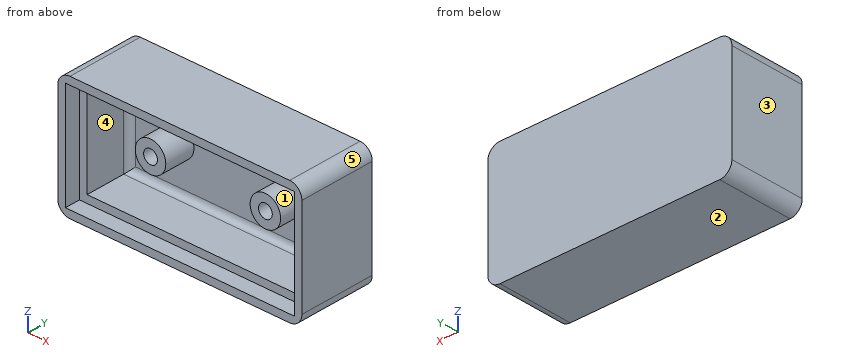
```python
from build123d import *

# Parameters (mm, degrees)
F0_W     = 50.8
F0_H     = 25.4
F0_W_2   = 44.45
F0_H_2   = 19.05
F1_DEPTH = 12.7
F2_W     = 44.45
F2_H     = 19.05
F3_DEPTH = 9.525
F4_R     = 1.27
F5_W     = 50.8
F5_H     = 25.4
F5_W_2   = 47.625
F5_H_2   = 22.225
F6_DEPTH = 3.175
F7_R     = 2.54
F8_R     = 3.175
F8_R_2   = 1.43697608
F9_DEPTH = 6.35


with BuildPart() as f1:
    # F0 (on Front) → F1 (new body)
    with BuildSketch(Plane.XZ):
        Rectangle(F0_W, F0_H)
        Rectangle(F0_W_2, F0_H_2, mode=Mode.SUBTRACT)
        Rectangle(F0_W_2, F0_H_2)
    extrude(amount=F1_DEPTH)

    # F2 (on face) → F3 (cut)
    with BuildSketch(Plane.XZ.offset(12.7)):
        Rectangle(F2_W, F2_H)
    extrude(amount=-F3_DEPTH, mode=Mode.SUBTRACT)

    # F4
    f4_edges = [f1.edges().sort_by_distance(p)[0] for p in [
        (22.225, -3.175, 0),
        (0, -3.175, 9.525),
        (-22.225, -3.175, 0),
        (0, -3.175, -9.525),
    ]]
    fillet(f4_edges, radius=F4_R)

    # F5 (on face) → F6 (join)
    with BuildSketch(Plane.XZ.offset(12.7)):
        Rectangle(F5_W, F5_H)
        Rectangle(F5_W_2, F5_H_2, mode=Mode.SUBTRACT)
    extrude(amount=F6_DEPTH)

    # F7
    f7_edges = [f1.edges().sort_by_distance(p)[0] for p in [
        (25.4, -7.9375, 12.7),
        (25.4, -7.9375, -12.7),
        (-25.4, -7.9375, -12.7),
        (-25.4, -7.9375, 12.7),
    ]]
    fillet(f7_edges, radius=F7_R)

    # F8 (on face) → F9 (join)
    with BuildSketch(Plane.XZ.offset(3.175)):
        with Locations((11.9508895849, 0)):
            Circle(F8_R)
        with Locations((11.9508895849, 0)):
            Circle(F8_R_2, mode=Mode.SUBTRACT)
        with Locations((-11.9508895849, 0)):
            Circle(F8_R)
        with Locations((-11.9508895849, 0)):
            Circle(F8_R_2, mode=Mode.SUBTRACT)
    extrude(amount=F9_DEPTH)


solid = f1.part
```
Work out the finished part from the listing and answer in its coordinate system (mm). Face numbers are marked on the shaded views. A direction names the side the tool comes from. Coordinates: 2 decimals unless noted, no trailing zeros. Write each loop counter-clockwise with the first axis right and the second up, starting at its lowest first coordinate (ties: lowest second). Pieces come first, ordered by that corner, then holes.
Q1. A cutting plane is placed at C-C, the plane x = -18. Give the vertices of the cut face in (y, z) (1 decimal), then the cut area to 3 significant figures.
Q2. Each of these flat-tipped pins is pushed along its axis until it touches: pin 1 Ø3 at (x, z) = (12.5, 0) entering from -Y (3 decimals); pin 2 Ø0.9 at (x, z) = (11.5, -0.5) entering from -Y (3 decimals). Where does it stop, or does it pass through?
Q3. Which of the six approach directions +Z, -Z, +X, -X, +Y, -Y give full straight-line access (tool end or side, diameter ignored) to the marked faces 4 and 5?
Q4. A cutting plane is placed at A-A, the plane y = -8. Give the vertices of the cut face in (x, z) (3 decimals).
Q5. Determine the mould class of the marked faces 1, 2 and 3 for opening direction X: released by +X, released by -X, zero draft, split by the parting line, or undercut.
Q6. A cutting plane is placed at D-D, the plane z = -5.5. Give the vertices of the cut face in (x, y) (1 decimal).
Q7. Find the intervals of material crossed by line 1 (Z direction, x = 4, y = -9.5) (3 decimals); line 2 (X direction, y = -9, z = -9) (3 decimals); line 3 (Z direction, x = 11.5, y = -9.25) (3 decimals), in increasing order.
Findings below:
1. outline: (-15.9, -12.7) - (0, -12.7) - (0, 12.7) - (-15.9, 12.7) - (-15.9, 11.1) - (-12.7, 11.1) - (-12.7, 9.5) - (-4.4, 9.5) arc R1.3 cw to (-3.2, 8.3) - (-3.2, -8.3) arc R1.3 cw to (-4.4, -9.5) - (-12.7, -9.5) - (-12.7, -11.1) - (-15.9, -11.1) - close
1. area: 152 mm2
2. pin 1: stops at y = -9.525
2. pin 2: stops at y = -3.175
3. face 4: -Y
3. face 5: +Z, +X, +Y, -Y
4. outline: (-25.4, -10.16) arc R2.54 ccw to (-22.86, -12.7) - (22.86, -12.7) arc R2.54 ccw to (25.4, -10.16) - (25.4, 10.16) arc R2.54 ccw to (22.86, 12.7) - (-22.86, 12.7) arc R2.54 ccw to (-25.4, 10.16) - close; circle Ø6.35 at (-11.951, 0); circle Ø6.35 at (11.951, 0); hole (-22.225, -9.525) - (22.225, -9.525) - (22.225, 9.525) - (-22.225, 9.525) - close; hole circle Ø2.874 at (-11.951, 0); hole circle Ø2.874 at (11.951, 0)
5. face 1: undercut
5. face 2: zero draft
5. face 3: released by -X
6. outline: (-25.4, -15.9) - (-23.8, -15.9) - (-23.8, -12.7) - (-22.2, -12.7) - (-22.2, -4.4) arc R1.3 cw to (-21, -3.2) - (21, -3.2) arc R1.3 cw to (22.2, -4.4) - (22.2, -12.7) - (23.8, -12.7) - (23.8, -15.9) - (25.4, -15.9) - (25.4, 0) - (-25.4, 0) - close
7. line 1: z = -12.7 to -9.525, 9.525 to 12.7
7. line 2: x = -25.4 to -22.225, 22.225 to 25.4
7. line 3: z = -12.7 to -9.525, -3.143 to -1.364, 1.364 to 3.143, 9.525 to 12.7
